Geometry check sheet. Reference: the model listing, model coordinates, mm. Face numbers are marked on the shaded views. A direction names the side the tool comes from. Round coordinates to 2 decimals unless told otherwise and drop trailing zeros. Write each loop counter-clockwise with the first axis right and the second up, starting at its lowest first coordinate (ties: lowest second). Pieces come first, ordered by that corner, then holes. Notation, with made-up numbers: (65.5, 19) -> (83.5, 19) arc R30 cw to (83.5, 45) -> close; hole circle Ø7 at (-15.5, -11.5). An arc over 180 degrees is marked (long way). Put each result on its own line as item: value. Start each with the question number.
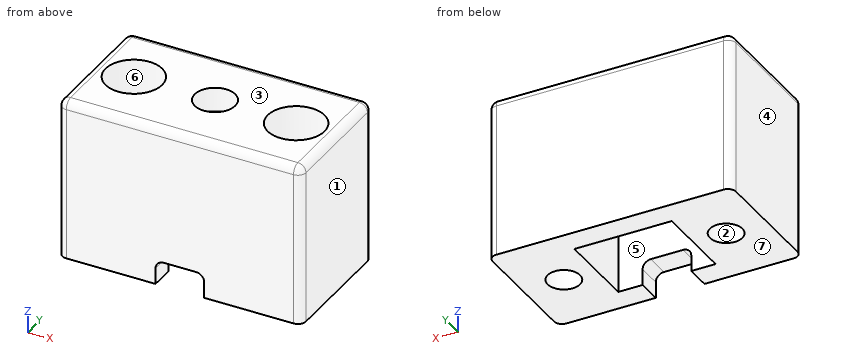
from build123d import *

# Parameters (mm, degrees)
BOX002_W          = 6
BOX002_H          = 10
BOX002_DEPTH      = 4
CYLINDER004_R     = 2.5
CYLINDER004_DEPTH = 10
CYLINDER_R        = 3.5
CYLINDER_DEPTH    = 33
CHAMFER_SIZE      = 3
CYLINDER001_R     = 3.5
CYLINDER001_DEPTH = 33
CHAMFER001_SIZE   = 3
CYLINDER002_R     = 2
CYLINDER002_DEPTH = 33
CYLINDER003_R     = 2
CYLINDER003_DEPTH = 33
BOX001_W          = 12
BOX001_H          = 10
BOX001_DEPTH      = 20
BOX_W             = 30
BOX_H             = 16
BOX_DEPTH         = 20
FILLET_R          = 1
FILLET001_R       = 1


with BuildPart() as cube002:
    # Box002 → Box002 (new body)
    with BuildSketch(Plane(origin=(12, -4, -1), x_dir=(1, 0, 0), z_dir=(0, 0, 1))):
        with Locations((3, 5)):
            Rectangle(BOX002_W, BOX002_H)
    extrude(amount=BOX002_DEPTH)


with BuildPart() as cylinder004:
    # Cylinder004 → Cylinder004 (new body)
    with BuildSketch(Plane(origin=(15, 8, 15), x_dir=(1, 0, 0), z_dir=(0, 0, 1))):
        Circle(CYLINDER004_R)
    extrude(amount=CYLINDER004_DEPTH)


with BuildPart() as chamfer_body:
    # Cylinder → Cylinder (new body)
    with BuildSketch(Plane(origin=(5, 8, -1), x_dir=(1, 0, 0), z_dir=(0, 0, 1))):
        Circle(CYLINDER_R)
    extrude(amount=CYLINDER_DEPTH)

    # Chamfer
    chamfer_edges = [chamfer_body.edges().sort_by_distance(p)[0] for p in [
        (1.5, 8, -1),
    ]]
    chamfer(chamfer_edges, length=CHAMFER_SIZE)


with BuildPart() as chamfer_body_1:
    # Chamfer placement: moved
    add(chamfer_body.part.moved(Location((0, 0, 4))))


with BuildPart() as chamfer001:
    # Cylinder001 → Cylinder001 (new body)
    with BuildSketch(Plane(origin=(25, 8, -1), x_dir=(1, 0, 0), z_dir=(0, 0, 1))):
        Circle(CYLINDER001_R)
    extrude(amount=CYLINDER001_DEPTH)

    # Chamfer001
    chamfer001_edges = [chamfer001.edges().sort_by_distance(p)[0] for p in [
        (21.5, 8, -1),
    ]]
    chamfer(chamfer001_edges, length=CHAMFER001_SIZE)


with BuildPart() as chamfer001_1:
    # Chamfer001 placement: moved
    add(chamfer001.part.moved(Location((0, 0, 4))))


with BuildPart() as cylinder002:
    # Cylinder002 → Cylinder002 (new body)
    with BuildSketch(Plane(origin=(5, 8, -1), x_dir=(1, 0, 0), z_dir=(0, 0, 1))):
        Circle(CYLINDER002_R)
    extrude(amount=CYLINDER002_DEPTH)


with BuildPart() as cylinder003:
    # Cylinder003 → Cylinder003 (new body)
    with BuildSketch(Plane(origin=(25, 8, -1), x_dir=(1, 0, 0), z_dir=(0, 0, 1))):
        Circle(CYLINDER003_R)
    extrude(amount=CYLINDER003_DEPTH)


with BuildPart() as holes:
    # Box001 → Box001 (new body)
    with BuildSketch(Plane(origin=(9, 3, -3), x_dir=(1, 0, 0), z_dir=(0, 0, 1))):
        with Locations((6, 5)):
            Rectangle(BOX001_W, BOX001_H)
    extrude(amount=BOX001_DEPTH)

    # Fusion: union Chamfer body, Chamfer001, Cylinder002, Cylinder003
    add(chamfer_body_1.part)
    add(chamfer001_1.part)
    add(cylinder002.part)
    add(cylinder003.part)


with BuildPart() as fillet001:
    # Box → Box (new body)
    with BuildSketch(Plane.XY):
        with Locations((15, 8)):
            Rectangle(BOX_W, BOX_H)
    extrude(amount=BOX_DEPTH)

    # Cut: cut holes
    add(holes.part, mode=Mode.SUBTRACT)

    # Cut001: cut Cylinder004
    add(cylinder004.part, mode=Mode.SUBTRACT)

    # Cut002: cut Cube002
    add(cube002.part, mode=Mode.SUBTRACT)

    # Fillet
    fillet_edges = [fillet001.edges().sort_by_distance(p)[0] for p in [
        (12, 1.5, 3),
        (18, 1.5, 3),
    ]]
    fillet(fillet_edges, radius=FILLET_R)

    # Fillet001
    fillet001_edges = [fillet001.edges().sort_by_distance(p)[0] for p in [
        (0, 0, 10),
        (15, 0, 20),
        (30, 0, 10),
        (0, 8, 20),
        (0, 16, 10),
        (30, 8, 20),
        (15, 16, 20),
        (30, 16, 10),
    ]]
    fillet(fillet001_edges, radius=FILLET001_R)


solid = fillet001.part
(1) Material ranges on L1, parallel to X at y = 8, z = 2.25; L2, parallel to Y at x = 5, z = 1.5; L3, parallel to X at y = 11, z = 15.25, recorded low to high. Write a range as from..to.
(2) Sectioned sample at D-D (z = 1.5). Record the cut outline in (x, y).
(3) Mould release check, pull along X, two halves, no side actions. Record for the marked faces 1, 2, 3 and 4: +X half, -X half, draft (parallel to the pull), parting line (faces both ways), or undercut.
(4) Sectioned sample at A-A (z = 17.5). Record the cut outline in (x, y).
(5) Sectioned sample at B-B (x = 15). Record the cut outline in (y, z).
(6) Set-up check for the marked faces 5, 6 and 7: record each of +Z, -Z, +X, -X, +Y, -Y from which the full face is reachable in a straight line by a thin tool's end or side.
(7) Sectioned sample at C-C (y = 8). State how many separate pieces and enclosed holes the cut face has, and give its area (3 significant figures).
(8) Go/stop test with flat-tipped pins: pin 1 Ø3.5 at (x, y) = (25, 8) entering from +Z; pin 2 Ø3.5 at (x, y) = (15.5, 2) entering from -Z. Record where each tip stops, or that it passes through.
Found:
1. L1: 0..3, 7..9, 21..23, 27..30
1. L2: 0..6, 10..16
1. L3: 0..3.2, 6.8..9, 21..23.2, 26.8..30
2. outline: (0, 1) arc R1 ccw to (1, 0) -> (12, 0) -> (12, 3) -> (9, 3) -> (9, 13) -> (21, 13) -> (21, 3) -> (18, 3) -> (18, 0) -> (29, 0) arc R1 ccw to (30, 1) -> (30, 15) arc R1 ccw to (29, 16) -> (1, 16) arc R1 ccw to (0, 15) -> close; hole circle Ø4 at (5, 8); hole circle Ø4 at (25, 8)
3. face 1: +X half
3. face 2: undercut
3. face 3: draft
3. face 4: -X half
4. outline: (0, 1) arc R1 ccw to (1, 0) -> (29, 0) arc R1 ccw to (30, 1) -> (30, 15) arc R1 ccw to (29, 16) -> (1, 16) arc R1 ccw to (0, 15) -> close; hole circle Ø7 at (5, 8); hole circle Ø5 at (15, 8); hole circle Ø7 at (25, 8)
5. outline: (0, 3) -> (3, 3) -> (3, 17) -> (5.5, 17) -> (5.5, 20) -> (1, 20) arc R1 ccw to (0, 19) -> close; (10.5, 17) -> (13, 17) -> (13, 0) -> (16, 0) -> (16, 19) arc R1 ccw to (15, 20) -> (10.5, 20) -> close
6. face 5: -Z
6. face 6: +Z
6. face 7: -Z, +X, -X, +Y, -Y
7. separate pieces: 4
7. enclosed holes: 0
7. area: 132 mm2
8. pin 1: through
8. pin 2: z = 2.97
